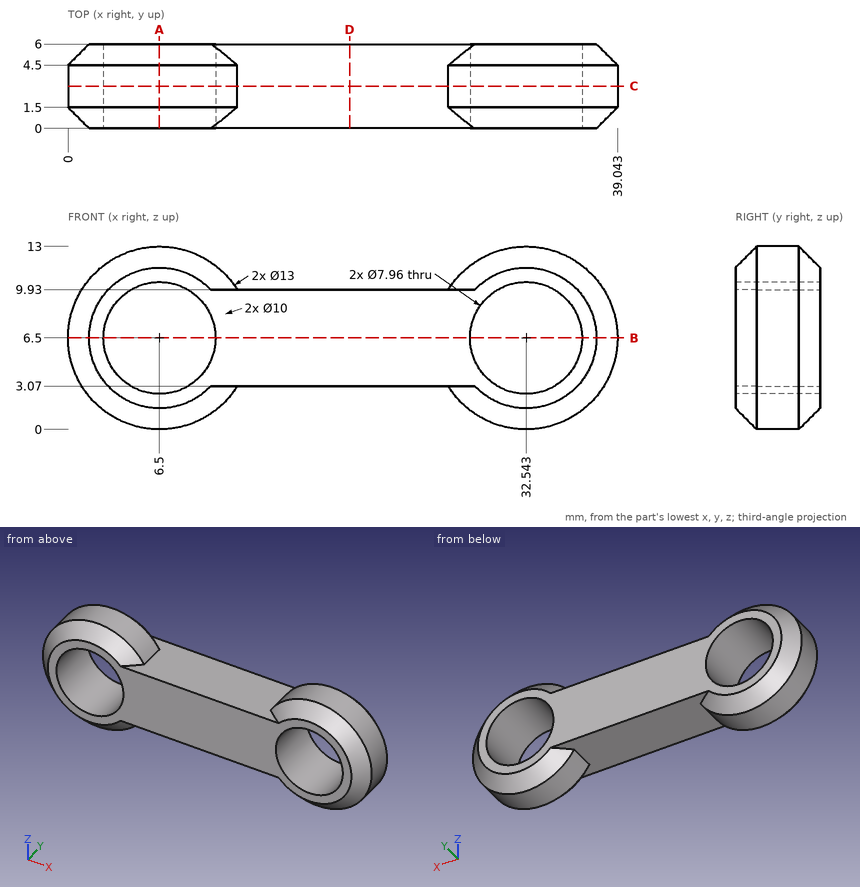
For this review, use the dimensioned drawing (mm, ordinates from the lowest corner) and the shaded views. Coordinates: 2 decimals unless noted, no trailing zeros. Write each loop counter-clockwise with the first axis right and the second up, starting at its lowest first coordinate (ties: lowest second). Pieces come first, ordered by that corner, then holes. Notation, with made-up numbers: (78.5, 9.25) -> (134.5, 9.25) arc R20 cw to (134.5, 26.25) -> close; hole circle Ø8 at (-5, 76). An arc over 180 degrees is marked (long way). Put each result on its own line as item: value.
Q1. Take a section at C-C, the plane y = 3. State the section outline as (x, z) points.
From the geometry:
outline: (12.02, 3.07) -> (27.02, 3.07) arc R6.5 ccw (long way) to (27.02, 9.93) -> (12.02, 9.93) arc R6.5 ccw (long way) to start; hole circle Ø7.96 at (6.5, 6.5); hole circle Ø7.96 at (32.54, 6.5)
Q2. Clearance check with flat-ended pins moving along their axes: pin 1 Ø3 at (x, y) = (21.5, 3) entering from -Z; pin 2 Ø1.5 at (x, z) = (28.5, 2) entering from -Y. State where each tip first meets the part, or that it passes through.
From the geometry:
pin 1: stops at z = 3.07
pin 2: stops at y = 0.3
Q3. Take a section at B-B, the plane z = 6.5. State the section outline as (x, y) points.
From the geometry:
outline: (0, 1.5) -> (1.5, 0) -> (2.52, 0) -> (2.52, 6) -> (1.5, 6) -> (0, 4.5) -> close; (10.48, 0) -> (28.56, 0) -> (28.56, 6) -> (10.48, 6) -> close; (36.52, 0) -> (37.54, 0) -> (39.04, 1.5) -> (39.04, 4.5) -> (37.54, 6) -> (36.52, 6) -> close
Q4. Take a section at A-A, the plane x = 6.5. State the section outline as (y, z) points.
From the geometry:
outline: (0, 1.5) -> (1.5, 0) -> (4.5, 0) -> (6, 1.5) -> (6, 2.52) -> (0, 2.52) -> close; (0, 10.48) -> (6, 10.48) -> (6, 11.5) -> (4.5, 13) -> (1.5, 13) -> (0, 11.5) -> close
Q5. Wall thickness on L1, parallel to X at y = 2.65, z = 6.5; L2, parallel to X at y = 5, z = 8.75 (1 decimal); L3, parallel to Z at x = 12.5, y = 2: over which ranges is each line inside the solid? List them lowest first.
From the geometry:
L1: x = 0 to 2.52, 10.48 to 28.56, 36.52 to 39.04
L2: x = 0.9 to 3.2, 9.8 to 29.3, 35.8 to 38.1
L3: z = 3.07 to 9.93
Q6. Take a section at D-D, the plane x = 20. State the section outline as (y, z) points.
From the geometry:
outline: (0, 3.07) -> (6, 3.07) -> (6, 9.93) -> (0, 9.93) -> close
